```python
from build123d import *

# Parameters (mm, degrees)
F0_R             = 8
F1_DEPTH         = 6
F3_DEPTH         = 2
F4_R             = 2
F5_DEPTH         = 1
F7_R             = 5.5
F8_DEPTH         = 22
F9_R             = 6.5
F9_R_2           = 5.5
F10_DEPTH        = 10
F11_SIZE         = 1
F12_W            = 1
F12_H            = 2
F13_DEPTH        = 20
F13_COPIES_COUNT = 10


# Not quite as in the source:
# - a fillet or chamfer that OpenCascade refuses, or shapes differently, is made with other operations: its cross-section is extruded or revolved along the edge and cut away or added
# - a pattern or mirror of a feature is missing from the dataset's text; its kind, count and spacing are read off the source's solid


with BuildPart() as f1:
    # F0 (on Front) → F1 (new body)
    with BuildSketch(Plane.XZ):
        Circle(F0_R)
    extrude(amount=-F1_DEPTH)

    # F2 (on face) → F3 (join)
    with BuildSketch(Plane.XZ):
        Polygon((1.7320508076, 3), (-1.7320508076, 3), (-3.4641016151, 0), (-1.7320508076, -3), (1.7320508076, -3), (3.4641016151, 0), align=None)
    extrude(amount=F3_DEPTH)

    # F4 (on face) → F5 (join)
    with BuildSketch(Plane.XZ.offset(2)):
        Circle(F4_R)
    extrude(amount=F5_DEPTH)

    # F6: fillet of radius 2 on 1 edges, made by hand

    # F6_s1 → F6_t2 (revolve, cut)
    with BuildSketch(Plane.XY):
        with BuildLine():
            ThreePointArc((2, -2), (1.2679491924, -2.7320508076), (0.2679491924, -3))
            Line((0.2679491924, -3), (2, -3))
            Line((2, -3), (2, -2))
        make_face()
    revolve(axis=Axis((0, -3, 0), (0, -1, 0)), mode=Mode.SUBTRACT)

    # F7 (on face) → F8 (join)
    with BuildSketch(Plane(origin=(0, 6, 0), x_dir=(-1, 0, 0), z_dir=(0, 1, 0))):
        Circle(F7_R)
    extrude(amount=F8_DEPTH)

    # F9 (on face) → F10 (join)
    with BuildSketch(Plane(origin=(0, 28, 0), x_dir=(-1, 0, 0), z_dir=(0, 1, 0))):
        Circle(F9_R)
        Circle(F9_R_2, mode=Mode.SUBTRACT)
    extrude(amount=-F10_DEPTH)

    # F11
    f11_edges = [f1.edges().sort_by_distance(p)[0] for p in [
        (6.5, 28, 0),
    ]]
    chamfer(f11_edges, length=F11_SIZE)

    # F12 (on face) → F13 (cut)
    with BuildSketch(Plane(origin=(0, 28, 0), x_dir=(-1, 0, 0), z_dir=(0, 1, 0))):
        with Locations((0, 6.7)):
            Rectangle(F12_W, F12_H)
    f13 = extrude(amount=-F13_DEPTH, mode=Mode.SUBTRACT)

    # F13_copies: F13 ×10 about axis
    f13_copies_axis = Axis((0, 0, 0), (0, 1, 0))
    for i in range(1, F13_COPIES_COUNT):
        add(f13.rotate(f13_copies_axis, i * 360 / F13_COPIES_COUNT), mode=Mode.SUBTRACT)


solid = f1.part
```
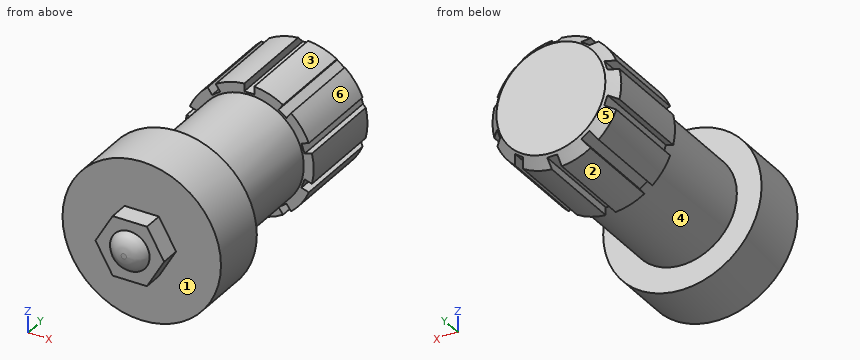
For this review, take the finished solid that the model builds, in its own axes (mm). Face numbers are marked on the shaded views. A direction names the side the tool comes from. Round coordinates to 2 decimals unless told otherwise and drop trailing zeros. Write each loop counter-clockwise with the first axis right and the second up, starting at its lowest first coordinate (ties: lowest second). Pieces come first, ordered by that corner, then holes. Notation, with made-up numbers: (82, 46.25) -> (135, 46.25) arc R15 cw to (135, 73.25) -> close; hole circle Ø9 at (-9, 13). An arc over 180 degrees is marked (long way). One line per question, with ' | ' between items. Start each with the question number.
(1) Tool access review of the marked faces 1, 2 and 3: name each direction out of +Z, -Z, +X, -X, +Y, -Y from which nothing blocks a thin tool from reaching the whole face with its end or side.
(2) Add section A-A, the plane y = -1. Write out the cut boundary in (x, z).
(3) Insertion check: P1, Ø4, axis at x = 2.5, y = 22.5, coming from the +Z side; P2, Ø0.8, axis at x = 0, y = 22, coming from the +Z side; P3, Ø0.6, axis at x = 0.5, y = -1.5, coming from the +Z side. Each pin has a flat end and moves straight along its axis. Give the tip position at first contact, or say it passes through.
(4) For line 1 along Y through (x, z) = (-7, -2); line 2 along Y through (x, z) = (1.25, -4.25); line 3 along Z through (x, y) = (4.75, 22), list the stretches that pass through material, from the lowest coordinate up. Write a range as from..to.
(5) Add section B-B, the plane y = 17. Write out the cut boundary in (x, z), plus the area to 3 significant figures.
(6) Mouldability with a two-part tool opening along Y and no side actions: class the marked faces 4, 5 and 6 as released by +Y, released by -Y, zero draft, split by the parting line, or undercut.
Answer list:
1) face 1: -Y | face 2: -Z, -X, +Y | face 3: +Z, +X, +Y
2) outline: (-3.46, 0) -> (-1.73, -3) -> (1.73, -3) -> (3.46, 0) -> (1.73, 3) -> (-1.73, 3) -> close
3) P1: z = 6.48 | P2: z = 5.7 | P3: z = 3
4) line 1: 0..6 | line 2: 0..28 | line 3: -4.44..4.44
5) outline: circle Ø11 at (0, 0) | area: 95.0 mm²
6) face 4: undercut | face 5: released by +Y | face 6: zero draft
